from build123d import *

# Parameters (mm, degrees)
SKETCH2_W               = 45
SKETCH2_H               = 49
BOSS_EXTRUDE1_DEPTH     = 1.5
CUT_EXTRUDE1_DEPTH      = 34.297897832
CUT_EXTRUDE1_DEPTH_BACK = 34.297897832
SKETCH3_R               = 1


with BuildPart() as part:
    # Sketch2 → Boss-Extrude1 (new body)
    with BuildSketch(Plane.XY):
        Rectangle(SKETCH2_W, SKETCH2_H)
    extrude(amount=BOSS_EXTRUDE1_DEPTH)

    # Sketch3 → Cut-Extrude1 (cut, two sides: drawn at the far end of the back side and taken through both)
    with BuildSketch(Plane.XY.offset(1.5).offset(-CUT_EXTRUDE1_DEPTH_BACK)):
        with Locations((-18.75, 20.75)):
            Circle(SKETCH3_R)
        with Locations(Location((18.75, 20.75, 0), (0, 0, 180))):
            Circle(SKETCH3_R)
        with Locations((18.75, -20.75)):
            Circle(SKETCH3_R)
        with Locations(Location((-18.75, -20.75, 0), (0, 0, 180))):
            Circle(SKETCH3_R)
    extrude(amount=CUT_EXTRUDE1_DEPTH + CUT_EXTRUDE1_DEPTH_BACK, mode=Mode.SUBTRACT)


solid = part.part
Input: part model. Units: mm. Frame: model coordinates. Give positions to 0.01 mm unless a question says otherwise; leave off trailing zeros. Write each loop counter-clockwise with the first axis right and the second up, starting at its lowest first coordinate (ties: lowest second). Pieces come first, ordered by that corner, then holes. Notation, with made-up numbers: M 8.25,59.5 L 23.25,59.5 A26 ccw 23.25,85.5 Z; hole C -32.5,81.25 d2. An arc over 180 degrees is marked long. Write item = value, one per line. Start each with the question number.
1) Cut plane B-B on y = -20.75. Return the cut outline in (x, z).
2) Cut plane A-A on x = 18.75. Return the cut outline in (y, z).
3) Draft query along X for faces 1 (the cylindrical face through (-18.967, 19.774, 0.739)), 2 (the flat face through (-22.5, 0, 1)), 3 (the flat face through (22.5, 0, 1)). Return one class per face: +X half, -X half, draft (parallel to the pull), parting line (faces both ways), or undercut.
4) Material intervals for line 1 along Y through (x, z) = (18.75, 0.6), sorted ascending. Write a range as [from, to].
Solved:
q1.outline = M -22.5,0 L -19.75,0 L -19.75,1.5 L -22.5,1.5 Z; M -17.75,0 L 17.75,0 L 17.75,1.5 L -17.75,1.5 Z; M 19.75,0 L 22.5,0 L 22.5,1.5 L 19.75,1.5 Z
q2.outline = M -24.5,0 L -21.75,0 L -21.75,1.5 L -24.5,1.5 Z; M -19.75,0 L 19.75,0 L 19.75,1.5 L -19.75,1.5 Z; M 21.75,0 L 24.5,0 L 24.5,1.5 L 21.75,1.5 Z
q3.face_1 = undercut
q3.face_2 = -X half
q3.face_3 = +X half
q4.line_1 = [-24.5, -21.75], [-19.75, 19.75], [21.75, 24.5]
